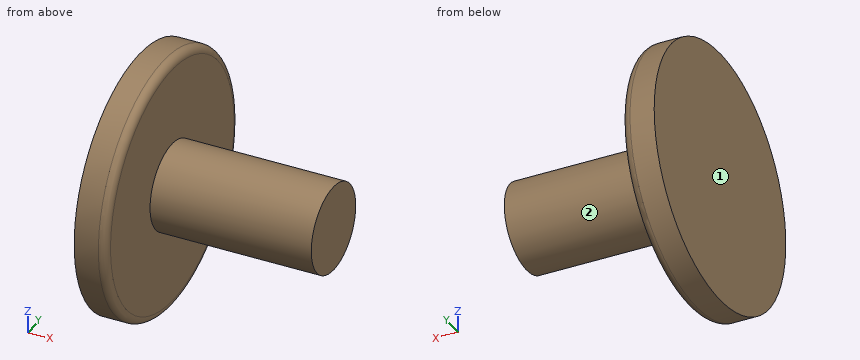
```python
from build123d import *

# Parameters (mm, degrees)
F0_R     = 8
F1_DEPTH = 2
F2_R     = 2.7
F3_DEPTH = 10
F4_R     = 0.5


with BuildPart() as f1:
    # F0 (on Right) → F1 (new body)
    with BuildSketch(Plane.YZ):
        with Locations((-26.541635, 17.838527)):
            Circle(F0_R)
    extrude(amount=F1_DEPTH)

    # F2 (on face) → F3 (join)
    with BuildSketch(Plane.YZ.offset(2)):
        with Locations((-26.541635, 17.838527)):
            Circle(F2_R)
    extrude(amount=F3_DEPTH)

    # F4
    f4_edges = [f1.edges().sort_by_distance(p)[0] for p in [
        (2, -34.541635, 17.838527),
    ]]
    fillet(f4_edges, radius=F4_R)


solid = f1.part
```
CAD build for the part. Positions are in the model's coordinates, mm. Face numbers are marked on the shaded views. A direction names the side the tool comes from. Round coordinates to 2 decimals unless told otherwise and drop trailing zeros. Loops run counter-clockwise (first coordinate to the right, second up) from the corner with the lowest first, then second, coordinate; pieces in that order, holes last. Notation, with made-up numbers: (70.25, 13.5) - (124.25, 13.5) arc R13 ccw to (124.25, 24.5) - close; hole circle Ø4 at (-37, 81.25). An arc over 180 degrees is marked (long way). Return JSON: item names as keys, results as strings. Group by question number.
Q1. Flat gauge pins, fed straight in: pin 1 Ø5 at (x, z) = (9.5, 19) entering from +Y; pin 2 Ø1 at (y, z) = (-29.5, 20) entering from -X; pin 3 Ø1.5 at (x, z) = (2, 15.5) entering from +Y; pin 4 Ø1 at (x, y) = (2, -20.5) entering from -Z. Where does each tip first touch, or does it go through?
Q2. Band-saw the part on A-A on x = 3. Give the cut face in (y, z).
Q3. Drill centre lines: line 1 along Z through (x, y) = (10.5, -26.5); line 2 along X through (y, z) = (-22.75, 11.75); line 3 along Y through (x, z) = (0.5, 17.75). Where is each one in solid material? Low to high. Write a range as [from, to].
Q4. Tool access for the marked faces 1 and 2: list every direction of +Z, -Z, +X, -X, +Y, -Y with a clear straight run to the whole face (end or side of a thin tool).
Solutions:
{
 "1": {"pin 1": "stops at y = -23.84", "pin 2": "stops at x = 0", "pin 3": "stops at y = -18.73", "pin 4": "stops at z = 12.22"},
 "2": {"outline": "circle Ø5.4 at (-26.54, 17.84)"},
 "3": {"line 1": "z = [15.14, 20.54]", "line 2": "x = [0, 2]", "line 3": "y = [-34.54, -18.54]"},
 "4": {"face 1": "+Z, -Z, -X, +Y, -Y", "face 2": "+X"}
}
